```python
from build123d import *

# Parameters (mm, degrees)
F1_DEPTH = 3.175


with BuildPart() as f1:
    # F0 (on Top) → F1 (new body)
    with BuildSketch(Plane.XY):
        with BuildLine():
            Line((-42.959198, -79.375), (-42.959198, -101.6))
            Line((-42.959198, -101.6), (-14.659364, -101.6))
            Line((-14.659364, -101.6), (-14.353896, -101.6))
            Line((-14.353896, -101.6), (-14.353896, -98.425))
            Line((-14.353896, -98.425), (-13.463448, -98.425))
            Line((-13.463448, -98.425), (11.046104, -98.425))
            Line((11.046104, -98.425), (11.046104, -101.6))
            Line((11.046104, -101.6), (11.936552, -101.6))
            Line((11.936552, -101.6), (14.022917, -101.6))
            Line((14.022917, -101.6), (39.525854, -101.6))
            Line((39.525854, -101.6), (39.651407, -101.6))
            Line((39.651407, -101.6), (39.651407, 101.6))
            Line((39.651407, 101.6), (14.022917, 101.6))
            Line((14.022917, 101.6), (13.768917, 101.6))
            Line((13.768917, 101.6), (11.936552, 101.6))
            Line((11.936552, 101.6), (11.046104, 101.6))
            Line((11.046104, 101.6), (11.046104, 98.425))
            Line((11.046104, 98.425), (-0.763448, 98.425))
            Line((-0.763448, 98.425), (-13.463448, 98.425))
            Line((-13.463448, 98.425), (-14.353896, 98.425))
            Line((-14.353896, 98.425), (-14.353896, 101.6))
            Line((-14.353896, 101.6), (-14.913364, 101.6))
            Line((-14.913364, 101.6), (-42.959198, 101.6))
            Line((-42.959198, 101.6), (-42.959198, 90.4875))
            ThreePointArc((-42.959198, 90.4875), (-7.018182, 5.55625), (-42.959198, -79.375))
        make_face()
    extrude(amount=F1_DEPTH)


solid = f1.part
```
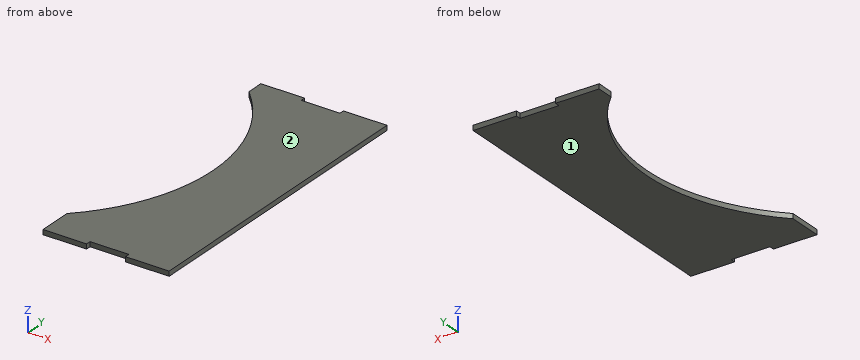
CAD build for the part. Positions are in the model's coordinates, mm. Face numbers are marked on the shaded views. Coordinates: 2 decimals unless noted, no trailing zeros. Order: outer loops, then holes, each group sorted by start corner. A loop starts at its lowest first (then second) coordinate and runs counter-clockwise, first axis right, second up. Notation, with made-up numbers: (29, -17.75) - (50, -17.75) arc R20 cw to (50, 11.25) - close; hole circle Ø1 at (-24, 22.25). An arc over 180 degrees is marked (long way). Answer in a Markdown table with one row per item.
1. Drill centre lines: L1, parallel to Y at x = -1, z = 1.1 (3 decimals); L2, parallel to Y at x = -22, z = 1.15; L3, parallel to Y at x = -26, z = 0.2. Where is each one in solid material? Low to high. Write a range as from..to.
Answer:
| item | result |
|---|---|
| L1 | -98.425..98.425 |
| L2 | -101.6..-52.07, 63.18..101.6 |
| L3 | -101.6..-58.72, 69.83..101.6 |
2. Slice it at D-D, the plane y = 16. List the corners of the cut face in (x, z) (3 decimals), then the cut area to 3 significant figures.
Answer:
| item | result |
|---|---|
| outline | (-7.48, 0) - (39.651, 0) - (39.651, 3.175) - (-7.48, 3.175) - close |
| area | 150 mm² |
3. Slice it at A-A, the plane x = -33. List the corners of the cut face in (y, z) (3 decimals), then the cut area to 3 significant figures.
Answer:
| item | result |
|---|---|
| outline | (-101.6, 0) - (-68.425, 0) - (-68.425, 3.175) - (-101.6, 3.175) - close; (79.538, 0) - (101.6, 0) - (101.6, 3.175) - (79.538, 3.175) - close |
| area | 175 mm² |
4. Pull direction Z, two halves, no side cores. Call the marked faces 1 and 2: +Z half, -Z half, draft (parallel to the pull), parting line (faces both ways), or undercut.
Answer:
| item | result |
|---|---|
| face 1 | -Z half |
| face 2 | +Z half |
5. Slice it at C-C, the plane x = -20.5. List the corners of the cut face in (y, z) (3 decimals).
Answer:
| item | result |
|---|---|
| outline | (-101.6, 0) - (-49.294, 0) - (-49.294, 3.175) - (-101.6, 3.175) - close; (60.407, 0) - (101.6, 0) - (101.6, 3.175) - (60.407, 3.175) - close |
6. Slice it at B-B, the plane z = 2.25. List the corners of the cut face in (x, y) (1 decimal).
Answer:
| item | result |
|---|---|
| outline | (-43, -101.6) - (-14.4, -101.6) - (-14.4, -98.4) - (11, -98.4) - (11, -101.6) - (39.7, -101.6) - (39.7, 101.6) - (11, 101.6) - (11, 98.4) - (-14.4, 98.4) - (-14.4, 101.6) - (-43, 101.6) - (-43, 90.5) arc R118.3 cw to (-43, -79.4) - close |
7. Flat gauge pin, fed straight in: P1, Ø1.6, axis at x = -4, z = 1.5, coming from the -Y side (3 decimals). Where does the tip first touch, or does it go through?
Answer:
| item | result |
|---|---|
| P1 | y = -98.425 |
